from build123d import *

# Parameters (mm, degrees)
F1_DEPTH      = 50.8
F1_DEPTH_BACK = 50.8
F2_R          = 5.08
F0_W          = 25.4
F0_H          = 25.4
F3_DEPTH      = 25.4
F3_DEPTH_BACK = 25.4


with BuildPart() as f1:
    # F0 (on Front) → F1 (new body, two sides)
    with BuildSketch(Plane.XZ) as f1_sk:
        Polygon((-65.414091, 25.4), (-65.414091, 0), (61.585909, 0), (61.585909, 25.4), (36.185909, 25.4), (-8.589925, 25.4), align=None)
    extrude(amount=F1_DEPTH)
    extrude(f1_sk.sketch, amount=-F1_DEPTH_BACK)

    # F2
    f2_edges = [f1.edges().sort_by_distance(p)[0] for p in [
        (61.585909, -50.8, 12.7),
        (61.585909, 50.8, 12.7),
        (-65.414091, 50.8, 12.7),
        (-65.414091, -50.8, 12.7),
    ]]
    fillet(f2_edges, radius=F2_R)

    # F0 (on Front) → F3 (join, two sides)
    with BuildSketch(Plane.XZ) as f3_sk:
        Polygon((-65.414091, 25.4), (-65.414091, 0), (61.585909, 0), (61.585909, 25.4), (36.185909, 25.4), (-8.589925, 25.4), align=None)
        with BuildLine():
            add(Edge.make_bspline(
                [(31.575521, 69.937845), (-10.358958, 69.028149), (-58.26536, 60.43693), (-65.414091, 25.4)],
                knots=[17.572505, 17.572505, 17.572505, 17.572505, 125.043548, 125.043548, 125.043548, 125.043548], degree=3))
            Line((-65.414091, 25.4), (-8.589925, 25.4))
            ThreePointArc((-8.589925, 25.4), (2.934524, 55.387008), (31.575521, 69.937845))
        make_face()
        with Locations((48.885909, 38.1)):
            Rectangle(F0_W, F0_H)
        with BuildLine():
            ThreePointArc((31.575521, 69.937845), (2.934524, 55.387008), (-8.589925, 25.4))
            Line((-8.589925, 25.4), (36.185909, 25.4))
            Line((36.185909, 25.4), (36.185909, 50.8))
            Line((36.185909, 50.8), (36.185909, 69.85))
            Line((36.185909, 69.85), (51.462281, 69.85))
            add(Edge.make_bspline(
                [(51.462281, 69.85), (45.129207, 70.029965), (38.432194, 70.086589), (31.575521, 69.937845)],
                knots=[0, 0, 0, 0, 17.572505, 17.572505, 17.572505, 17.572505], degree=3))
        make_face()
        Polygon((36.185909, 50.8), (61.585909, 50.8), (112.385909, 50.8), (112.385909, 69.85), (51.462281, 69.85), (36.185909, 69.85), align=None)
    extrude(amount=F3_DEPTH)
    extrude(f3_sk.sketch, amount=-F3_DEPTH_BACK)


solid = f1.part
Check sheet for the modelled part. Datum: model origin and axes. Units: mm. A direction names the side the tool comes from. Give positions to 0.01 mm unless a question says otherwise; leave off trailing zeros. Loops run counter-clockwise (first coordinate to the right, second up) from the corner with the lowest first, then second, coordinate; pieces in that order, holes last. Notation, with made-up numbers: M 76.25,50 L 131.25,50 A36 ccw 131.25,85 Z; hole C 31.5,15.25 d10. An arc over 180 degrees is marked long. Answer as a JSON object with one key per item and string values. Group by question number.
Q1. Go/stop test with flat-tipped pins: P1, Ø1.5, axis at x = 88, y = -18, coming from the +Z side; P2, Ø4, axis at x = 4.5, y = 8.5, coming from the +Z side; P3, Ø12, axis at y = 12, z = 44.5, coming from the +X side. Record where each tip stops, or that it passes through.
Q2. Cross-section at B-B on y = 34.5. Record the cut outline in (x, z), then the cut area to 3 significant figures.
Q3. Cross-section at A-A on z = 23. Record the cut outline in (x, y).
Q4. Access from +Z, -Z, +X, -X, +Y, -Y to the whole of each face (thin tool, end or side, straight path). Record for faces 1 (the flat face through (82, 0, 69.85)), 2 (the flat face through (61.586, -1, 19)), 3 (the flat face through (22, 25.4, 48)), 4 (the flat face through (22, -25.4, 48)), 5 (the cylindrical face through (60.14, 49.27, 12.88)).
Q5. Cross-section at C-C on x = 97. Record the cut outline in (y, z), then the cut area to 3 significant figures.
Q6. Material ranges on line 1 along Y through (x, z) = (9, 52); line 2 along X through (y, z) = (-38, 24.5); line 3 along Z through (x, y) = (14, 35.5), recorded low to high. Write a range as [from, to].
Evaluation:
{
 "1": {"P1": "stops at z = 69.85", "P2": "stops at z = 68.37", "P3": "stops at x = 61.59"},
 "2": {"outline": "M -65.41,0 L 61.59,0 L 61.59,25.4 L -65.41,25.4 Z", "area": "3,230 mm2"},
 "3": {"outline": "M -65.41,-45.72 A5.08 ccw -60.33,-50.8 L 56.51,-50.8 A5.08 ccw 61.59,-45.72 L 61.59,45.72 A5.08 ccw 56.51,50.8 L -60.33,50.8 A5.08 ccw -65.41,45.72 Z"},
 "4": {"face 1": "+Z, +X, +Y, -Y", "face 2": "-Z, +X, +Y, -Y", "face 3": "+Z, +X, -X, +Y", "face 4": "+Z, +X, -X, -Y", "face 5": "+Z, -Z, +X, +Y"},
 "5": {"outline": "M -25.4,50.8 L 25.4,50.8 L 25.4,69.85 L -25.4,69.85 Z", "area": "968 mm2"},
 "6": {"line 1": "y = [-25.4, 25.4]", "line 2": "x = [-65.41, 61.59]", "line 3": "z = [0, 25.4]"}
}
